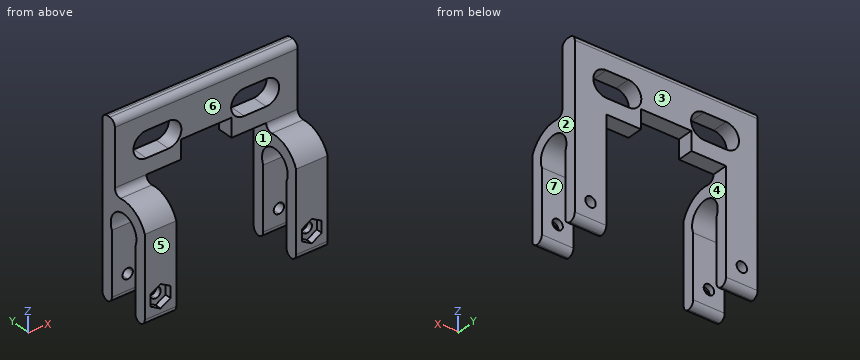
from build123d import *

# Parameters (mm, degrees)
F1_DEPTH     = 17
F3_DEPTH     = 80
F4_T4_DEPTH  = 16.4862536334
F4_T10_DEPTH = 10
F4_T15_DEPTH = 10
F4_T20_DEPTH = 10
F4_T25_DEPTH = 10
F4_T30_DEPTH = 16.4862536334
F4_T33_DEPTH = 68
F4_T35_DEPTH = 20
F4_T37_DEPTH = 20
F5_R         = 1.65
F6_DEPTH     = 2


# Not quite as in the source:
# - a fillet or chamfer that OpenCascade refuses, or shapes differently, is made with other operations: its cross-section is extruded or revolved along the edge and cut away or added


with BuildPart() as f1:
    # F0 (on Front) → F1 (new body)
    with BuildSketch(Plane.XZ):
        Polygon((-13, 18.9721025527), (-13, -25), (-8, -25), (-3, -25), (-3, -5), (-3, 0), (-3, 5), (-3, 10), (8, 10), (8, 16), (24, 16), (24, 10), (35, 10), (35, 5), (35, 0), (35, -5), (35, -25), (40, -25), (45, -25), (45, 25), (45, 30), (-13, 30), (-13, 25), align=None)
        Polygon((-4.9, -19.7897858345), (-8, -21.579571669), (-11.1, -19.7897858345), (-11.1, -16.2102141655), (-8, -14.420428331), (-4.9, -16.2102141655), align=None, mode=Mode.SUBTRACT)
        Polygon((43.1, -19.7897858345), (40, -21.579571669), (36.9, -19.7897858345), (36.9, -16.2102141655), (40, -14.420428331), (43.1, -16.2102141655), align=None, mode=Mode.SUBTRACT)
        with BuildLine():
            ThreePointArc((-3, 14.8721025527), (-7.1, 18.9721025527), (-3, 23.0721025527))
            Line((-3, 23.0721025527), (4, 23.0721025527))
            ThreePointArc((4, 23.0721025527), (8.1, 18.9721025527), (4, 14.8721025527))
            Line((4, 14.8721025527), (-3, 14.8721025527))
        make_face(mode=Mode.SUBTRACT)
        with BuildLine():
            ThreePointArc((28, 14.8721025527), (23.9, 18.9721025527), (28, 23.0721025527))
            Line((28, 23.0721025527), (35, 23.0721025527))
            ThreePointArc((35, 23.0721025527), (39.1, 18.9721025527), (35, 14.8721025527))
            Line((35, 14.8721025527), (28, 14.8721025527))
        make_face(mode=Mode.SUBTRACT)
        Polygon((36.9, -19.7897858345), (40, -21.579571669), (43.1, -19.7897858345), (43.1, -16.2102141655), (40, -14.420428331), (36.9, -16.2102141655), align=None)
        with BuildLine():
            ThreePointArc((41.65, -18), (41.166726189, -19.166726189), (40, -19.65))
            ThreePointArc((40, -19.65), (38.833273811, -16.833273811), (41.65, -18))
        make_face(mode=Mode.SUBTRACT)
        Polygon((-11.1, -19.7897858345), (-8, -21.579571669), (-4.9, -19.7897858345), (-4.9, -16.2102141655), (-8, -14.420428331), (-11.1, -16.2102141655), align=None)
        with BuildLine():
            ThreePointArc((-6.35, -18), (-6.833273811, -19.166726189), (-8, -19.65))
            ThreePointArc((-8, -19.65), (-9.166726189, -16.833273811), (-6.35, -18))
        make_face(mode=Mode.SUBTRACT)
    extrude(amount=F1_DEPTH)

    # F2 (on face) → F3 (cut)
    with BuildSketch(Plane.YZ.offset(45)):
        with BuildLine():
            Line((-17, 30), (-17, 2.3871079109))
            ThreePointArc((-17, 2.3871079109), (-12.0593125845, 7.429341251), (-5, 7.4541409972))
            Line((-5, 7.4541409972), (-5, 30))
            Line((-5, 30), (-17, 30))
        make_face()
        with BuildLine():
            Line((-3.8, -25), (-3.8, -3.1053503271))
            ThreePointArc((-3.8, -3.1053503271), (-8.5, 4.15), (-13.2, -3.1053503271))
            Line((-13.2, -3.1053503271), (-13.2, -25))
            Line((-13.2, -25), (-4, -25))
            Line((-4, -25), (-3.8, -25))
        make_face()
    extrude(amount=-F3_DEPTH, mode=Mode.SUBTRACT)

    # F4: fillet of radius 2 on 12 edges, made by hand


with BuildPart() as f4_tool2:
    # F4_s3 → F4_t4 (new body)
    with BuildSketch(Plane.YZ.offset(3.4862536334)):
        with BuildLine():
            ThreePointArc((-5, 10.0486424505), (-5.6843474227, 8.5423030811), (-7.269058296, 8.0668231769))
            ThreePointArc((-7.269058296, 8.0668231769), (-6.1147752276, 7.8336404039), (-5, 7.4541409972))
            Line((-5, 7.4541409972), (-5, 10.0486424505))
        make_face()
    extrude(amount=-F4_T4_DEPTH)

    split(bisect_by=Plane.YZ.offset(-3), keep=Keep.TOP)

    split(bisect_by=Plane.XY.offset(10), keep=Keep.TOP)


with BuildPart() as f1_1:
    add(f1.part)

    # F4_t1: union F4_tool2
    add(f4_tool2.part)


with BuildPart() as f4_tool8:
    # F4_s9 → F4_t10 (new body)
    with BuildSketch(Plane.YZ.offset(-3)):
        with BuildLine():
            ThreePointArc((-5, 10.0486424505), (-5.6843474227, 8.5423030811), (-7.269058296, 8.0668231769))
            ThreePointArc((-7.269058296, 8.0668231769), (-6.1147752276, 7.8336404039), (-5, 7.4541409972))
            Line((-5, 7.4541409972), (-5, 10.0486424505))
        make_face()
    extrude(amount=-F4_T10_DEPTH)

    split(bisect_by=Plane.XY.offset(10), keep=Keep.TOP)


with BuildPart() as f1_2:
    add(f1_1.part)

    # F4_t7: union F4_tool8
    add(f4_tool8.part)


with BuildPart() as f4_tool13:
    # F4_s14 → F4_t15 (new body)
    with BuildSketch(Plane.YZ.offset(-3)):
        with BuildLine():
            ThreePointArc((-5, 10.0486424505), (-5.6843474227, 8.5423030811), (-7.269058296, 8.0668231769))
            ThreePointArc((-7.269058296, 8.0668231769), (-6.1147752276, 7.8336404039), (-5, 7.4541409972))
            Line((-5, 7.4541409972), (-5, 10.0486424505))
        make_face()
    extrude(amount=-F4_T15_DEPTH)

    split(bisect_by=Plane.XY.offset(10), keep=Keep.BOTTOM)


with BuildPart() as f1_3:
    add(f1_2.part)

    # F4_t12: union F4_tool13
    add(f4_tool13.part)


with BuildPart() as f4_tool18:
    # F4_s19 → F4_t20 (new body)
    with BuildSketch(Plane.YZ.offset(45)):
        with BuildLine():
            ThreePointArc((-5, 10.0486424505), (-5.6843474227, 8.5423030811), (-7.269058296, 8.0668231769))
            ThreePointArc((-7.269058296, 8.0668231769), (-6.1147752276, 7.8336404039), (-5, 7.4541409972))
            Line((-5, 7.4541409972), (-5, 10.0486424505))
        make_face()
    extrude(amount=-F4_T20_DEPTH)

    split(bisect_by=Plane.XY.offset(10), keep=Keep.TOP)


with BuildPart() as f1_4:
    add(f1_3.part)

    # F4_t17: union F4_tool18
    add(f4_tool18.part)


with BuildPart() as f4_tool23:
    # F4_s24 → F4_t25 (new body)
    with BuildSketch(Plane.YZ.offset(45)):
        with BuildLine():
            ThreePointArc((-5, 10.0486424505), (-5.6843474227, 8.5423030811), (-7.269058296, 8.0668231769))
            ThreePointArc((-7.269058296, 8.0668231769), (-6.1147752276, 7.8336404039), (-5, 7.4541409972))
            Line((-5, 7.4541409972), (-5, 10.0486424505))
        make_face()
    extrude(amount=-F4_T25_DEPTH)

    split(bisect_by=Plane.XY.offset(10), keep=Keep.BOTTOM)


with BuildPart() as f1_5:
    add(f1_4.part)

    # F4_t22: union F4_tool23
    add(f4_tool23.part)


with BuildPart() as f4_tool28:
    # F4_s29 → F4_t30 (new body)
    with BuildSketch(Plane.YZ.offset(45)):
        with BuildLine():
            ThreePointArc((-5, 10.0486424505), (-5.6843474227, 8.5423030811), (-7.269058296, 8.0668231769))
            ThreePointArc((-7.269058296, 8.0668231769), (-6.1147752276, 7.8336404039), (-5, 7.4541409972))
            Line((-5, 7.4541409972), (-5, 10.0486424505))
        make_face()
    extrude(amount=-F4_T30_DEPTH)

    split(bisect_by=Plane.XY.offset(10), keep=Keep.TOP)

    split(bisect_by=Plane.YZ.offset(35), keep=Keep.BOTTOM)


with BuildPart() as f1_6:
    add(f1_5.part)

    # F4_t27: union F4_tool28
    add(f4_tool28.part)

    # F4_s34 → F4_t33 (cut)
    with BuildSketch(Plane.YZ.offset(-18)):
        with BuildLine():
            ThreePointArc((-5, 28), (-4.4142135624, 29.4142135624), (-3, 30))
            Line((-3, 30), (-5, 30))
            Line((-5, 30), (-5, 28))
        make_face()
        with BuildLine():
            ThreePointArc((-2, 30), (-0.5857864376, 29.4142135624), (0, 28))
            Line((0, 28), (0, 30))
            Line((0, 30), (-2, 30))
        make_face()
    extrude(amount=F4_T33_DEPTH, mode=Mode.SUBTRACT)

    # F4_s36 → F4_t35 (cut)
    with BuildSketch(Plane.YZ.offset(30)):
        with BuildLine():
            ThreePointArc((-15, -25), (-16.4142135624, -24.4142135624), (-17, -23))
            Line((-17, -23), (-17, -25))
            Line((-17, -25), (-15, -25))
        make_face()
        with BuildLine():
            ThreePointArc((-13.2, -23), (-13.7857864376, -24.4142135624), (-15.2, -25))
            Line((-15.2, -25), (-13.2, -25))
            Line((-13.2, -25), (-13.2, -23))
        make_face()
        with BuildLine():
            ThreePointArc((-1.8, -25), (-3.2142135624, -24.4142135624), (-3.8, -23))
            Line((-3.8, -23), (-3.8, -25))
            Line((-3.8, -25), (-1.8, -25))
        make_face()
        with BuildLine():
            ThreePointArc((-2, -25), (-0.5857864376, -24.4142135624), (0, -23))
            Line((0, -23), (0, -25))
            Line((0, -25), (-2, -25))
        make_face()
    extrude(amount=F4_T35_DEPTH, mode=Mode.SUBTRACT)

    # F4_s38 → F4_t37 (cut)
    with BuildSketch(Plane.YZ.offset(-18)):
        with BuildLine():
            ThreePointArc((-15, -25), (-16.4142135624, -24.4142135624), (-17, -23))
            Line((-17, -23), (-17, -25))
            Line((-17, -25), (-15, -25))
        make_face()
        with BuildLine():
            ThreePointArc((-13.2, -23), (-13.7857864376, -24.4142135624), (-15.2, -25))
            Line((-15.2, -25), (-13.2, -25))
            Line((-13.2, -25), (-13.2, -23))
        make_face()
        with BuildLine():
            ThreePointArc((-1.8, -25), (-3.2142135624, -24.4142135624), (-3.8, -23))
            Line((-3.8, -23), (-3.8, -25))
            Line((-3.8, -25), (-1.8, -25))
        make_face()
        with BuildLine():
            ThreePointArc((-2, -25), (-0.5857864376, -24.4142135624), (0, -23))
            Line((0, -23), (0, -25))
            Line((0, -25), (-2, -25))
        make_face()
    extrude(amount=F4_T37_DEPTH, mode=Mode.SUBTRACT)

    # F5 (on face) → F6 (cut)
    with BuildSketch(Plane.XZ.offset(17)):
        Polygon((-4.85, -19.8186533479), (-4.85, -16.1813466521), (-8, -14.3626933041), (-11.15, -16.1813466521), (-11.15, -19.8186533479), (-8, -21.6373066959), align=None)
        with Locations((-8, -18)):
            Circle(F5_R, mode=Mode.SUBTRACT)
        Polygon((36.85, -16.1813466521), (36.85, -19.8186533479), (40, -21.6373066959), (43.15, -19.8186533479), (43.15, -16.1813466521), (40, -14.3626933041), align=None)
    extrude(amount=-F6_DEPTH, mode=Mode.SUBTRACT)


solid = f1_6.part
The model under review builds one solid part; all positions refer to its coordinate system, in mm. Face numbers are marked on the shaded views. A direction names the side the tool comes from. Give positions to 0.01 mm unless a question says otherwise; leave off trailing zeros. Loops run counter-clockwise (first coordinate to the right, second up) from the corner with the lowest first, then second, coordinate; pieces in that order, holes last. Notation, with made-up numbers: (75, 83) -> (128, 83) arc R24 ccw to (128, 106) -> close; hole circle Ø9 at (-11.75, 9). An arc over 180 degrees is marked (long way). Put each result on its own line as item: value. Start each with the question number.
1. For the marked faces 5, 6 and 7, list the 3-axis set-ups (+Z, -Z, +X, -X, +Y, -Y) from which the entire face can be reached by the end or side of a thin tool; tool diameter is ignored.
2. Mouldability with a two-part tool opening along X and no side actions: class the marked faces 1, 2, 3 and 4 as released by +X, released by -X, zero draft, split by the parting line, or undercut.
3. We need section B-B on x = 32.5. State the section outline as (y, z) points, then the cut area to 3 significant figures.
4. Clearance check with flat-ended pins moving along their axes: P1, Ø3, axis at x = 38.5, y = -14, coming from the +Z side; P2, Ø20, axis at x = 5.5, z = 17.5, coming from the -Y side; P3, Ø4, axis at x = 32.5, y = -3, coming from the -Z side. State where each tip first meets the part, or that it passes through.
5. We need section C-C on y = -8.5. State the section outline as (x, z) points.
6. Wall thickness on probe 1 along X at (y, z) = (-13.6, -18); probe 2 along X at (y, z) = (-15.25, 1.5); probe 3 along Y at (x, z) = (-10, -9): over which ranges is each line inside the solid? List them lowest first.
7. We need section A-A on z = -5. State the section outline as (x, y) points.
8. We need section D-D on z = 6.5. State the section outline as (x, y) points, then the cut area to 3 significant figures.
Determined:
1. face 5: +Z, -Z, +X, -X, -Y
1. face 6: +Z, +X, -X, -Y
1. face 7: -Z, +X, -X
2. face 1: undercut
2. face 2: released by +X
2. face 3: zero draft
2. face 4: undercut
3. outline: (-5, 10) -> (0, 10) -> (0, 14.87) -> (-5, 14.87) -> (-5, 10.05) arc R2 cw to start; (-5, 23.07) -> (0, 23.07) -> (0, 28) arc R2 ccw to (-2, 30) -> (-3, 30) arc R2 ccw to (-5, 28) -> close
3. area: 57.3 mm^2
4. P1: z = 7.23
4. P2: y = -5
4. P3: z = 10
5. outline: (-13, 4.15) -> (-3, 4.15) -> (-3, 8.15) -> (-13, 8.15) -> close; (35, 4.15) -> (45, 4.15) -> (45, 8.15) -> (35, 8.15) -> close
6. probe 1: -13 to -9.65, -6.35 to -3, 35 to 38.35, 41.65 to 45
6. probe 2: -13 to -3, 35 to 45
6. probe 3: -17 to -13.2, -3.8 to 0
7. outline: (-13, -17) -> (-3, -17) -> (-3, -13.2) -> (-13, -13.2) -> close; (-13, -3.8) -> (-3, -3.8) -> (-3, 0) -> (-13, 0) -> close; (35, -17) -> (45, -17) -> (45, -13.2) -> (35, -13.2) -> close; (35, -3.8) -> (45, -3.8) -> (45, 0) -> (35, 0) -> close
8. outline: (-13, -13.74) -> (-3, -13.74) -> (-3, 0) -> (-13, 0) -> close; (35, -13.74) -> (45, -13.74) -> (45, 0) -> (35, 0) -> close
8. area: 275 mm^2
